Build history of the part. All positions in model axes, mm. Face numbers are marked on the shaded views. A direction names the side the tool comes from. Coordinates: 2 decimals unless noted, no trailing zeros. Loops run counter-clockwise (first coordinate to the right, second up) from the corner with the lowest first, then second, coordinate; pieces in that order, holes last. Notation, with made-up numbers: (-7.75, -4) -> (-0.75, -4) arc R12 cw to (-0.75, 14) -> close; hole circle Ø3 at (55.25, -23). An arc over 180 degrees is marked (long way). One line per item, written item: value. Start each with the question number.
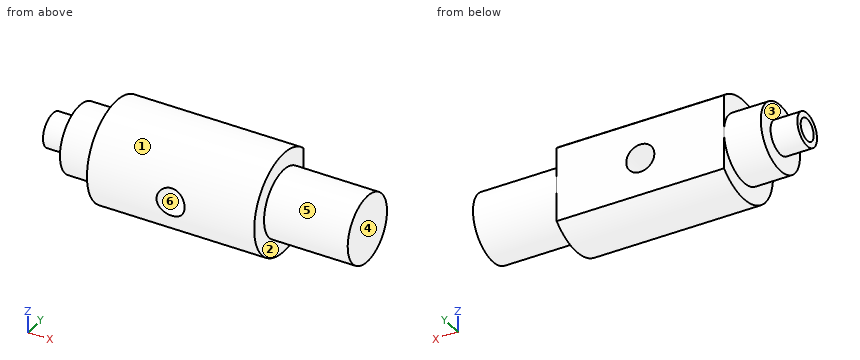
```python
from build123d import *

# Parameters (mm, degrees)
CUT_EXTRUDE_START        = 5
SKETCH_2_W               = 25
SKETCH_2_H               = 23.22226429
CUT_EXTRUDE_1_DEPTH      = 23.156951228
HOLE_WIZARD_M5_1_D       = 4.2
CUT_EXTRUDE_2_DEPTH      = 52.11262078
CUT_EXTRUDE_2_DEPTH_BACK = 7
SKETCH_6_OUTSIDE_W       = 27.736
SKETCH_6_OUTSIDE_H       = 25.236
SKETCH_6_OUTSIDE_R       = 2.5
CUT_EXTRUDE_START_2      = -3
SKETCH_7_R               = 2.5
CUT_EXTRUDE_3_DEPTH      = 3
HOLE_WIZARD_M4_1_D       = 3.3
HOLE_WIZARD_M4_1_DEPTH   = 8
HOLE_WIZARD_M4_1_TIP     = 0.991420021


with BuildPart() as part:
    # 草图1 → 旋转1 (revolve)
    with BuildSketch(Plane.XY, mode=Mode.PRIVATE) as revolve_1_sk:
        Polygon((0, 7.5), (12.5, 7.5), (12.5, 5), (25, 5), (25, 0), (0, 0), align=None)
    revolve_1 = revolve(revolve_1_sk.sketch.rotate(Axis((0, 0, 0), (1, 0, 0)), 90), axis=Axis((0, 0, 0), (1, 0, 0)))

    # 镜向1: 旋转1 across plane
    add(revolve_1.mirror(Plane(origin=(0, 0, 0), x_dir=(0, 0, 1), z_dir=(1, 0, 0))))

    # 草图2 → 切除-拉伸1 (cut, through all)
    with BuildSketch(Plane(origin=(0, 0, 0), x_dir=(1, 0, 0), z_dir=(0, 1, 0)).offset(CUT_EXTRUDE_START)):
        Rectangle(SKETCH_2_W, SKETCH_2_H)
    extrude(amount=CUT_EXTRUDE_1_DEPTH, mode=Mode.SUBTRACT)

    # M5 螺纹孔的螺纹孔钻头1 (through all)
    with Locations(Plane(origin=(0, 5, 0), x_dir=(1, 0, 0), z_dir=(0, 1, 0))):
        with Locations((0, 0)):
            Hole(HOLE_WIZARD_M5_1_D / 2)

    # 草图6 outside → 切除-拉伸2 (cut, two sides: drawn at the far end of the back side and taken through both)
    with BuildSketch(Plane.ZY.offset(25).offset(-CUT_EXTRUDE_2_DEPTH_BACK)):
        with Locations((0, -1.25)):
            Rectangle(SKETCH_6_OUTSIDE_W, SKETCH_6_OUTSIDE_H)
        with Locations(Location((0, 0, 0), (0, 0, 180))):
            Circle(SKETCH_6_OUTSIDE_R, mode=Mode.SUBTRACT)
    extrude(amount=CUT_EXTRUDE_2_DEPTH + CUT_EXTRUDE_2_DEPTH_BACK, mode=Mode.SUBTRACT)

    # 草图7 → 切除-拉伸3 (cut)
    with BuildSketch(Plane.ZY.offset(25).offset(CUT_EXTRUDE_START_2)):
        with Locations(Location((0, 0, 0), (0, 0, 180))):
            Circle(SKETCH_7_R)
    extrude(amount=CUT_EXTRUDE_3_DEPTH, mode=Mode.SUBTRACT)

    # M4 螺纹孔的螺纹孔钻头1
    with Locations(Plane.ZY.offset(22)):
        with Locations((0, 0)):
            Hole(HOLE_WIZARD_M4_1_D / 2, depth=HOLE_WIZARD_M4_1_DEPTH)
            with Locations((0, 0, -(HOLE_WIZARD_M4_1_DEPTH + HOLE_WIZARD_M4_1_TIP / 2))):  # 118° drill point
                Cone(0, HOLE_WIZARD_M4_1_D / 2, HOLE_WIZARD_M4_1_TIP, mode=Mode.SUBTRACT)


solid = part.part
```
Item 1: Band-saw the part on D-D, the plane z = 3.5. List the corners of the cut face in (x, y), and give its area (3 significant figures).
Item 2: Band-saw the part on A-A, the plane x = 0. List the corners of the cut face in (y, z).
Item 3: Drop flat-ended pins along their axis: pin 1 Ø6 at (x, z) = (-14, 1) entering from -Y; pin 2 Ø1.5 at (y, z) = (-5, -6) entering from +X; pin 3 Ø3 at (y, z) = (0, 0) entering from -X; pin 4 Ø6 at (x, y) = (19.5, -2) entering from +Z. Give the stop position or say it passes through.
Item 4: Two-plate mould, pull along X, no slides. Class the marked faces 4, 5 and 6: +X half, -X half, draft (parallel to the pull), parting line (faces both ways), or undercut.
Item 5: Band-saw the part on C-C, the plane x = -19. List the corners of the cut face in (y, z), and give its area (3 significant figures).
Item 6: Probe probe 1 along Y at (x, z) = (-18.5, 0); probe 2 along Y at (x, z) = (-16, 0); probe 3 along Z at (x, y) = (21, 0.25). List the from-to ranges inside material, lowest first.
Item 7: Tool access for the marked faces 1, 2 and 3: list every direction of +Z, -Z, +X, -X, +Y, -Y with a clear straight run to the whole face (end or side of a thin tool).
Item 8: Band-saw the part on B-B, the plane y = -6.5. List the corners of the cut face in (x, z).
Worked out:
1. outline: (-18, -3.57) -> (-12.5, -3.57) -> (-12.5, -6.63) -> (12.5, -6.63) -> (12.5, -3.57) -> (25, -3.57) -> (25, 3.57) -> (12.5, 3.57) -> (12.5, 5) -> (-12.5, 5) -> (-12.5, 3.57) -> (-18, 3.57) -> close
1. area: 419 mm²
2. outline: (-7.2, -2.1) arc R7.5 ccw to (5, -5.59) -> (5, -2.1) -> close; (-7.2, 2.1) -> (5, 2.1) -> (5, 5.59) arc R7.5 ccw to start
3. pin 1: stops at y = -7.5
3. pin 2: stops at x = 12.5
3. pin 3: stops at x = -13.91
3. pin 4: stops at z = 5
4. face 4: +X half
4. face 5: draft
4. face 6: undercut
5. outline: circle Ø5 at (0, 0); hole circle Ø3.3 at (0, 0)
5. area: 11.1 mm²
6. probe 1: y = -2.5 to -1.65, 1.65 to 2.5
6. probe 2: y = -5 to -1.65, 1.65 to 5
6. probe 3: z = -4.99 to 4.99
7. face 1: +X, -X
7. face 2: +X
7. face 3: -X
8. outline: (-12.5, -3.74) -> (12.5, -3.74) -> (12.5, 3.74) -> (-12.5, 3.74) -> close; hole circle Ø4.2 at (0, 0)
